from build123d import *

# Parameters (mm, degrees)
BOSS_EXTRUDE1_DEPTH     = 22.5
SKETCH3_R               = 1.75
CUT_EXTRUDE1_DEPTH      = 8
MIRROR3_COPY_1_SKETCH_R = 1.75
MIRROR3_COPY_1_DEPTH    = 8


with BuildPart() as part:
    # Sketch1 → Boss-Extrude1 (new, symmetric)
    with BuildSketch(Plane(origin=(0, 0, 0), x_dir=(0, 0, -1), z_dir=(1, 0, 0))):
        Polygon((5, -6), (5, -13.5), (-5, -13.5), (-5, 13.5), (5, 13.5), (5, 6), (0, 6), (0, -6), align=None)
    extrude(amount=BOSS_EXTRUDE1_DEPTH, both=True)

    # Sketch3 → Cut-Extrude1 (cut)
    with BuildSketch(Plane.XY.offset(5)):
        with Locations((-10, 10)):
            Circle(SKETCH3_R)
    cut_extrude1 = extrude(amount=-CUT_EXTRUDE1_DEPTH, mode=Mode.SUBTRACT)

    # Mirror2: Cut-Extrude1 across plane
    add(cut_extrude1.mirror(Plane.ZX), mode=Mode.SUBTRACT)

    # Mirror3: Cut-Extrude1 across plane
    add(cut_extrude1.mirror(Plane(origin=(0, 0, 0), x_dir=(0, 0, 1), z_dir=(1, 0, 0))), mode=Mode.SUBTRACT)

    # Mirror3 copy 1 sketch → Mirror3 copy 1 (cut)
    with BuildSketch(Plane(origin=(0, 0, 5), x_dir=(-1, 0, 0), z_dir=(0, 0, 1))):
        with Locations((-10, 10)):
            Circle(MIRROR3_COPY_1_SKETCH_R)
    extrude(amount=-MIRROR3_COPY_1_DEPTH, mode=Mode.SUBTRACT)


solid = part.part
Design review of the part built by this model. Coordinates are the model's own, in mm. A direction names the side the tool comes from. Round coordinates to 2 decimals unless told otherwise and drop trailing zeros. Write each loop counter-clockwise with the first axis right and the second up, starting at its lowest first coordinate (ties: lowest second). Pieces come first, ordered by that corner, then holes. Notation, with made-up numbers: (25, -1) -> (74, -1) arc R25 ccw to (74, 17) -> close; hole circle Ø8 at (-14.75, 19.5). An arc over 180 degrees is marked (long way). One line per item, written item: value. Start each with the question number.
Q1. Add section A-A (z = -3.5). Give the boundary of the cut face in (x, y), then the cut area to 3 significant figures.
Q2. To check wall thickness, follow probe 1 along Y at (x, z) = (10, 1.5); probe 2 along X at (y, z) = (-10, 1.5); probe 3 along Y at (x, z) = (-10, -0.25). State the ranges of each line that lie inside material, in increasing order.
Q3. Add section D-D (y = -10). Give the boundary of the cut face in (x, z).
Q4. Tool access review of faces 1 (the face through (0, -6, -2)), 2 (the face through (9.1, -11.5, 1.1)), 3 (the face through (0, 0, 5)): name each direction out of +Z, -Z, +X, -X, +Y, -Y from which nothing blocks a thin tool from reaching the whole face with its end or side.
Q5. Add section C-C (z = 1). Give the boundary of the cut face in (x, y), then the cut area to 3 significant figures.
Q6. Add section B-B (x = -10). Give the boundary of the cut face in (y, z).
Q7. The part is to be moulded in two halves that separate along Y. For faces 4 (the face through (10, 10, -3)), 5 (the face through (0, -13.5, 0)), 6 (the face through (22.5, 0, 1)), say which applies: pulls with the +Y half, pulls with the -Y half, needs draft (parallel to the pull), parting line crosses it, or undercut.
Q8. Insertion check: P1, Ø3, axis at x = -9.5, y = 9.5, coming from the +Z side; P2, Ø3, axis at x = 10, y = -10, coming from the +Z side. Each pin has a flat end and moves straight along its axis. Give the tip position at first contact, or say it passes through.
Response:
1. outline: (-22.5, -13.5) -> (22.5, -13.5) -> (22.5, -6) -> (-22.5, -6) -> close; (-22.5, 6) -> (22.5, 6) -> (22.5, 13.5) -> (-22.5, 13.5) -> close
1. area: 675 mm^2
2. probe 1: y = -13.5 to -11.75, -8.25 to 8.25, 11.75 to 13.5
2. probe 2: x = -22.5 to -11.75, -8.25 to 8.25, 11.75 to 22.5
2. probe 3: y = -13.5 to -11.75, -8.25 to -6, 6 to 8.25, 11.75 to 13.5
3. outline: (-22.5, -5) -> (22.5, -5) -> (22.5, 5) -> (11.75, 5) -> (11.75, -3) -> (8.25, -3) -> (8.25, 5) -> (-8.25, 5) -> (-8.25, -3) -> (-11.75, -3) -> (-11.75, 5) -> (-22.5, 5) -> close
4. face 1: -Z, +X, -X
4. face 2: +Z
4. face 3: +Z, +X, -X, +Y, -Y
5. outline: (-22.5, -13.5) -> (22.5, -13.5) -> (22.5, 13.5) -> (-22.5, 13.5) -> close; hole circle Ø3.5 at (-10, -10); hole circle Ø3.5 at (-10, 10); hole circle Ø3.5 at (10, -10); hole circle Ø3.5 at (10, 10)
5. area: 1,180 mm^2
6. outline: (-13.5, -5) -> (-6, -5) -> (-6, 0) -> (6, 0) -> (6, -5) -> (13.5, -5) -> (13.5, 5) -> (11.75, 5) -> (11.75, -3) -> (8.25, -3) -> (8.25, 5) -> (-8.25, 5) -> (-8.25, -3) -> (-11.75, -3) -> (-11.75, 5) -> (-13.5, 5) -> close
7. face 4: undercut
7. face 5: pulls with the -Y half
7. face 6: needs draft
8. P1: stops at z = 5
8. P2: stops at z = -3
